```python
from build123d import *

# Parameters (mm, degrees)
SKETCH1_R           = 5
SKETCH1_R_2         = 3.175
BOSS_EXTRUDE1_DEPTH = 12
SKETCH2_R           = 11
SKETCH2_R_2         = 3.175
BOSS_EXTRUDE2_DEPTH = 2.000000064
SKETCH3_R           = 1.5
CUT_EXTRUDE1_DEPTH  = 13
SKETCH4_R           = 1.500000048
CUT_EXTRUDE2_DEPTH  = 16.556349186


with BuildPart() as part:
    # Sketch1 → Boss-Extrude1 (new body)
    with BuildSketch(Plane(origin=(0, 0, 0), x_dir=(1, 0, 0), z_dir=(0, 1, 0))):
        Circle(SKETCH1_R)
        Circle(SKETCH1_R_2, mode=Mode.SUBTRACT)
    extrude(amount=BOSS_EXTRUDE1_DEPTH)

    # Sketch2 → Boss-Extrude2 (add)
    with BuildSketch(Plane(origin=(0, 12, 0), x_dir=(1, 0, 0), z_dir=(0, 1, 0))):
        Circle(SKETCH2_R)
        Circle(SKETCH2_R_2, mode=Mode.SUBTRACT)
    extrude(amount=-BOSS_EXTRUDE2_DEPTH)

    # Sketch3 → Cut-Extrude1 (cut, through all)
    with BuildSketch(Plane(origin=(0, 12, 0), x_dir=(1, 0, 0), z_dir=(0, 1, 0))):
        with Locations((0, 8)):
            Circle(SKETCH3_R)
        with Locations((8, 0)):
            Circle(SKETCH3_R)
        with Locations((0, -8)):
            Circle(SKETCH3_R)
        with Locations((-8, 0)):
            Circle(SKETCH3_R)
    extrude(amount=-CUT_EXTRUDE1_DEPTH, mode=Mode.SUBTRACT)

    # Sketch4 → Cut-Extrude2 (cut, through all)
    with BuildSketch(Plane(origin=(0, 0, 0), x_dir=(0, 1, 0), z_dir=(0.707106781, 0, 0.707106781))):
        with Locations((3.500000112, 0)):
            Circle(SKETCH4_R)
    extrude(amount=-CUT_EXTRUDE2_DEPTH, mode=Mode.SUBTRACT)


solid = part.part
```
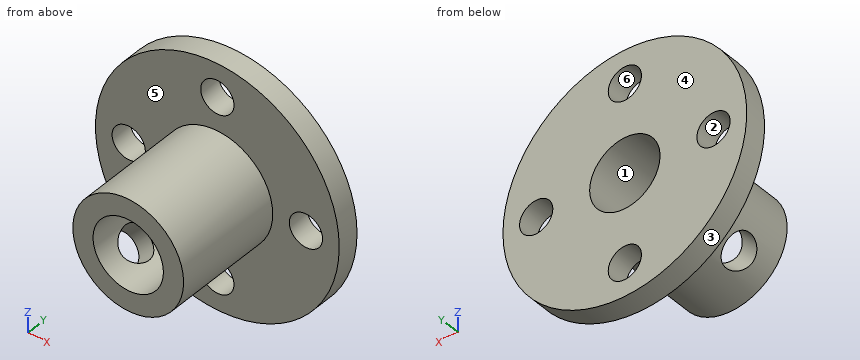
Work out the finished part from the listing and answer in its coordinate system (mm). Face numbers are marked on the shaded views. A direction names the side the tool comes from. Coordinates: 2 decimals unless noted, no trailing zeros. Loops run counter-clockwise (first coordinate to the right, second up) from the corner with the lowest first, then second, coordinate; pieces in that order, holes last. Notation, with made-up numbers: (17, 85.5) - (70, 85.5) arc R7 cw to (70, 97.5) - close; hole circle Ø1 at (65, 24.25). An arc over 180 degrees is marked (long way). Use a Markdown table: item, result.
Item 1: Find section B-B, the plane x = 0. Determine the outline of the cut face in (y, z) (3 decimals), and give its area (3 significant figures).
Evaluation:
| item | result |
|---|---|
| outline | (0, -5) - (10, -5) - (10, -6.5) - (12, -6.5) - (12, -3.175) - (0, -3.175) - close; (0, 3.175) - (12, 3.175) - (12, 6.5) - (10, 6.5) - (10, 5) - (0, 5) - close; (10, -11) - (12, -11) - (12, -9.5) - (10, -9.5) - close; (10, 9.5) - (12, 9.5) - (12, 11) - (10, 11) - close |
| area | 55.8 mm2 |
Item 2: Find section A-A, the plane z = 0. Determine the outline of the cut face in (x, y) (3 decimals).
Evaluation:
| item | result |
|---|---|
| outline | (-11, 10) - (-9.5, 10) - (-9.5, 12) - (-11, 12) - close; (-6.5, 10) - (-5, 10) - (-5, 0) - (-3.175, 0) - (-3.175, 12) - (-6.5, 12) - close; (3.175, 0) - (5, 0) - (5, 10) - (6.5, 10) - (6.5, 12) - (3.175, 12) - close; (9.5, 10) - (11, 10) - (11, 12) - (9.5, 12) - close |
Item 3: Consider probe 1 along X at (y, z) = (10.55, 0) (3 decimals); probe 2 along Z at (x, y) = (0, 4.75) (3 decimals). Determine where each line is inside the solid, lowest interval first. Write a range as from..to.
Evaluation:
| item | result |
|---|---|
| probe 1 | x = -11..-9.5, -6.5..-3.175, 3.175..6.5, 9.5..11 |
| probe 2 | z = -5..-3.175, 3.175..5 |
Item 4: Given pin 1 Ø5 at (x, z) = (1.5, 8) entering from -Y; pin 2 Ø4 at (y, z) = (2, 2.5) entering from -X; pin 3 Ø6 at (x, y) = (-4.5, 10.5) entering from -Z; pin 4 Ø4 at (x, z) = (0, 0) entering from +Y, each flat-ended and moving along its own axis, determine where each tip first touches the part or whether it passes through.
Evaluation:
| item | result |
|---|---|
| pin 1 | stops at y = 10 |
| pin 2 | stops at x = -4.97 |
| pin 3 | stops at z = -10.9 |
| pin 4 | passes through |
Item 5: Find section D-D, the plane y = 11. Determine the outline of the cut face in (x, z) (3 decimals), and give its area (3 significant figures).
Evaluation:
| item | result |
|---|---|
| outline | circle Ø22 at (0, 0); hole circle Ø3 at (-8, 0); hole circle Ø6.35 at (0, 0); hole circle Ø3 at (0, -8); hole circle Ø3 at (0, 8); hole circle Ø3 at (8, 0) |
| area | 320 mm2 |
Item 6: For the marked faces 5 and 6, determine the directions among +Z, -Z, +X, -X, +Y, -Y from which every point of the face is accessible in a straight line to the end or side of a thin tool.
Evaluation:
| item | result |
|---|---|
| face 5 | -Y |
| face 6 | +Y, -Y |
Item 7: The mould has two halves that part along Z. Classify the marked faces 1, 2, 3 and 4: +Z half, -Z half, draft (parallel to the pull), parting line (faces both ways), or undercut.
Evaluation:
| item | result |
|---|---|
| face 1 | undercut |
| face 2 | undercut |
| face 3 | parting line |
| face 4 | draft |
Item 8: Find section C-C, the plane z = 8. Determine the outline of the cut face in (x, y), and give its area (3 significant figures).
Evaluation:
| item | result |
|---|---|
| outline | (-7.55, 10) - (-1.5, 10) - (-1.5, 12) - (-7.55, 12) - close; (1.5, 10) - (7.55, 10) - (7.55, 12) - (1.5, 12) - close |
| area | 24.2 mm2 |
